Could you check a few things on this model? Use its own coordinates, in mm. Coordinates: 2 decimals unless noted, no trailing zeros. Loops run counter-clockwise (first coordinate to the right, second up) from the corner with the lowest first, then second, coordinate; pieces in that order, holes last. Notation, with made-up numbers: M -27.5,-28.5 L 21.5,-28.5 A21 cw 21.5,-9.5 Z; hole C 46.25,19 d8. An arc over 180 degrees is marked long. Return JSON: item names as keys, results as strings. Group by question number.
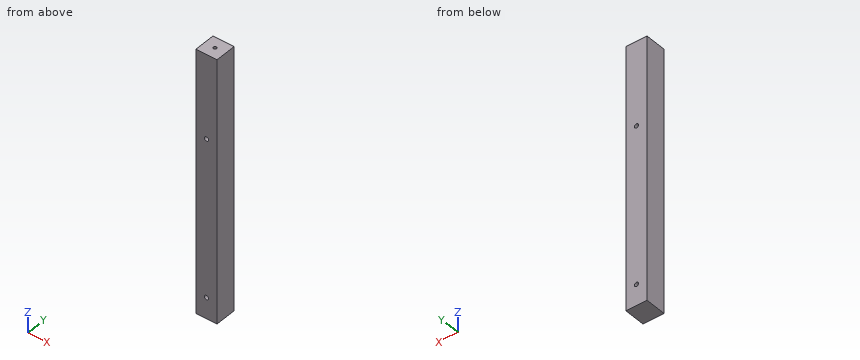
Autodesk Inventor part; units mm, degrees
ref_plane "YZ Plane" through (0, 0, 0) normal (1, 0, 0) x (0, 1, 0)
ref_plane "XZ Plane" through (0, 0, 0) normal (0, 1, 0) x (-1, 0, 0)
ref_plane "XY Plane" through (0, 0, 0) normal (0, 0, 1) x (1, 0, 0)
sketch "Sketch1" plane through (0, 0, 0) normal (0, 0, 1) x (1, 0, 0)
  line L0 (0, 0) -> (-20, 0)
  line L1 (-20, 0) -> (-20, 20)
  line L2 (-20, 20) -> (0, 20)
  line L3 (0, 20) -> (0, 0)
  dimension "d0" = 20
  dimension "d1" = 20
extrude "Extrusion1" add sketch "Sketch1" along normal blind 250
sketch "Sketch2" plane through (0, 0, 250) normal (0, 0, 1) x (1, 0, 0)
  line L0 (0, 0) -> (-20, 20) construction
  circle A0 centre (-10, 10) radius 1.5
  dimension "d4" = 3
extrude "Extrusion2" cut sketch "Sketch2" against normal blind 100
sketch "Sketch3" plane through (-20, 20, 0) normal (0, 1, 0) x (1, 0, 0)
  line L0 (20, 0) -> (0, 0)
  line L1 (10, 0) -> (10, -250) construction
  circle A0 centre (10, -20) radius 2
  circle A1 centre (10, -170) radius 2
  dimension "d7" = 4
  dimension "d8" = 4
  dimension "d9" = 20
  dimension "d11" = 150
extrude "Extrusion3" cut sketch "Sketch3" against normal through all
properties part number "legno 1" material "Wood (Birch)"
(1) Imagine slicing it at A-A, the plane z = 161.5. Write out the boundary of the cut face in (x, y).
(2) Will these pins go through, and if not, where does the flat tip stop? P1, Ø8, axis at x = -10, z = 79.5, coming from the -Y side; P2, Ø1.8, axis at x = -10, y = 10, coming from the +Z side.
(3) If I drill on L1, parallel to Z at x = -10, y = 16.25; L2, parallel to X at y = 10, z = 155; L3, parallel to Y at x = -10, z = 158, over which ranges is the centre line in solid material (lowest first)? Write a range as [from, to].
Checks:
{
 "1": {"outline": "M -20,0 L 0,0 L 0,20 L -20,20 Z; hole C -10,10 d3"},
 "2": {"P1": "y = 0", "P2": "z = 150"},
 "3": {"L1": "[0, 18], [22, 168], [172, 250]", "L2": "[-20, -11.5], [-8.5, 0]", "L3": "[0, 8.5], [11.5, 20]"}
}
